Design review of the part built by this model. Coordinates are the model's own, in mm. Face numbers are marked on the shaded views. Give positions to 0.01 mm unless a question says otherwise; leave off trailing zeros. Order: outer loops, then holes, each group sorted by start corner. A loop starts at its lowest first (then second) coordinate and runs counter-clockwise, first axis right, second up. Notation, with made-up numbers: (13.25, 51) -> (60.25, 51) arc R13 ccw to (60.25, 66) -> close; hole circle Ø11 at (63.5, 49). An arc over 180 degrees is marked (long way). One line per item, written item: value. Start each with the question number.
1) Consider section A-A (z = 2.25). State the section outline as (x, y) points, plus the area to 3 significant figures.
2) Consider section B-B (y = -39). State the section outline as (x, z) points.
3) Wall thickness on line 1 along X through (y, z) = (-42, 1.2); line 2 along Y through (x, z) = (-0.75, 1.45); line 3 along X through (y, z) = (5.5, 1.35): over which ranges is each line inside the solid? List them lowest first. Write a range as from..to.
4) The part is to be moulded in two halves that separate along Y. For the marked faces 1, 2, 3 and 4, say which applies: released by +Y, released by -Y, zero draft, split by the parting line, or undercut.
5) Consider section C-C (x = 7.25). State the section outline as (y, z) points, plus the area to 3 significant figures.
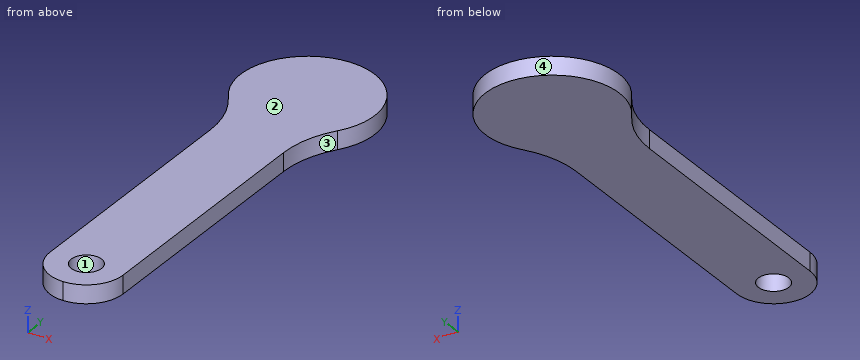
from build123d import *

# Parameters (mm, degrees)
SKETCH1_R           = 2.5
BOSS_EXTRUDE1_DEPTH = 3


with BuildPart() as part:
    # Sketch1 → Boss-Extrude1 (new body)
    with BuildSketch(Plane.XY):
        with BuildLine():
            Line((6.025139131, -15.636232903), (6.025139131, -57))
            ThreePointArc((6.025139131, -57), (4.260416737, -61.260416737), (0, -63.025139131))
            ThreePointArc((0, -63.025139131), (-4.260416737, -61.260416737), (-6.025139131, -57))
            Line((-6.025139131, -57), (-6.025139131, -15.636232903))
            ThreePointArc((-6.025139131, -15.636232903), (-6.781462516, -10.778273635), (-8.978839155, -6.380168449))
            ThreePointArc((-8.978839155, -6.380168449), (0, 11.014812844), (8.978839155, -6.380168449))
            ThreePointArc((8.978839155, -6.380168449), (6.781462516, -10.778273635), (6.025139131, -15.636232903))
        make_face()
        with Locations((0, -57)):
            Circle(SKETCH1_R, mode=Mode.SUBTRACT)
    extrude(amount=BOSS_EXTRUDE1_DEPTH)


solid = part.part
Checked values:
1. outline: (-8.98, -6.38) arc R15.98 cw to (-6.03, -15.64) -> (-6.03, -57) arc R6.03 ccw to (6.03, -57) -> (6.03, -15.64) arc R15.98 cw to (8.98, -6.38) arc R11.01 ccw (long way) to start; hole circle Ø5 at (0, -57)
1. area: 988 mm^2
2. outline: (-6.03, 0) -> (6.03, 0) -> (6.03, 3) -> (-6.03, 3) -> close
3. line 1: x = -6.03..6.03
3. line 2: y = -62.98..-59.38, -54.62..10.99
3. line 3: x = -9.54..9.54
4. face 1: undercut
4. face 2: zero draft
4. face 3: released by -Y
4. face 4: split by the parting line
5. outline: (-9.5, 0) -> (8.29, 0) -> (8.29, 3) -> (-9.5, 3) -> close
5. area: 53.4 mm^2
